from build123d import *

# Parameters (mm, degrees)
BOSS_EXTRUDE1_DEPTH = 30
SKETCH2_W           = 19.5
SKETCH2_H           = 19.5
BOSS_EXTRUDE2_DEPTH = 19.5
SKETCH3_W           = 55
SKETCH3_H           = 10
BOSS_EXTRUDE3_DEPTH = 2.5


with BuildPart() as part:
    # Sketch1 → Boss-Extrude1 (new body)
    with BuildSketch(Plane.XY):
        Polygon((12, 0), (12, 3), (5, 3), (5, 7), (50, 7), (50, 3), (43, 3), (43, 0), (55, 0), (55, 10), (0, 10), (0, 0), align=None)
    extrude(amount=BOSS_EXTRUDE1_DEPTH)

    # Sketch2 → Boss-Extrude2 (add)
    with BuildSketch(Plane(origin=(0, 10, 0), x_dir=(1, 0, 0), z_dir=(0, 1, 0))):
        with Locations((27.5, -15)):
            Rectangle(SKETCH2_W, SKETCH2_H)
    extrude(amount=BOSS_EXTRUDE2_DEPTH)

    # Sketch3 → Boss-Extrude3 (add)
    with BuildSketch(Plane(origin=(0, 0, 0), x_dir=(-1, 0, 0), z_dir=(0, 0, -1))):
        with Locations((-27.5, 5)):
            Rectangle(SKETCH3_W, SKETCH3_H)
    extrude(amount=BOSS_EXTRUDE3_DEPTH)


solid = part.part
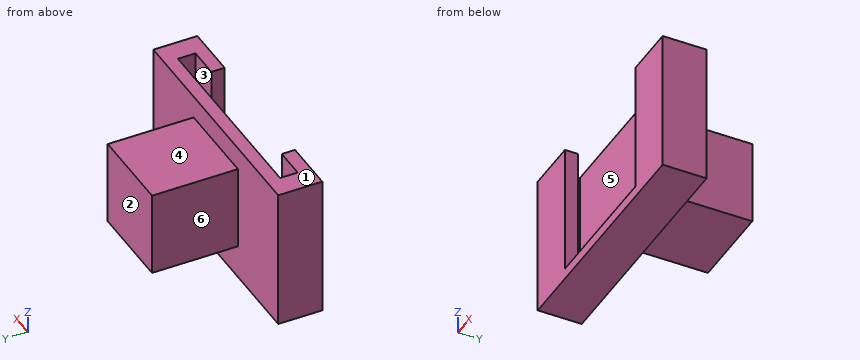
Read the model definition and answer for the solid it produces. Units are mm, in the model's axes. Face numbers are marked on the shaded views. A direction names the side the tool comes from. Round coordinates to 2 decimals unless told otherwise and drop trailing zeros. Write each loop counter-clockwise with the first axis right and the second up, starting at its lowest first coordinate (ties: lowest second). Pieces come first, ordered by that corner, then holes. Notation, with made-up numbers: (-24.5, 40.5) - (13.5, 40.5) arc R27 ccw to (13.5, 79.5) - close; hole circle Ø11 at (-9.75, 19). An arc over 180 degrees is marked (long way). Use a Markdown table: item, result.
(1) The part is cut by section A-A (x = 44). Write down the section's boundary in (y, z), then the cut area to 3 significant figures.
Reported:
| item | result |
|---|---|
| outline | (0, -2.5) - (10, -2.5) - (10, 30) - (7, 30) - (7, 0) - (3, 0) - (3, 30) - (0, 30) - close |
| area | 205 mm2 |
(2) Each of these flat-tipped pins is pushed along its axis until it touches: pin 1 Ø9 at (x, z) = (36, 20.5) entering from -Y; pin 2 Ø5.5 at (x, y) = (23, 2) entering from +Z; pin 3 Ø5 at (x, y) = (35.5, 18.5) entering from +Z. Where does it stop, or does it pass through?
Reported:
| item | result |
|---|---|
| pin 1 | y = 7 |
| pin 2 | z = 0 |
| pin 3 | z = 24.75 |
(3) The part is cut by section C-C (z = 4). Write down the section's boundary in (x, y).
Reported:
| item | result |
|---|---|
| outline | (0, 0) - (12, 0) - (12, 3) - (5, 3) - (5, 7) - (50, 7) - (50, 3) - (43, 3) - (43, 0) - (55, 0) - (55, 10) - (0, 10) - close |
(4) Which of the six approach directions +Z, -Z, +X, -X, +Y, -Y give full straight-line access (tool end or side, diameter ignored) to the marked faces 4, 5 and 6?
Reported:
| item | result |
|---|---|
| face 4 | +Z, +X, -X, +Y |
| face 5 | +Z |
| face 6 | +Z, -Z, -X, +Y |
(5) The mould has two halves that part along Y. Classify the marked faces 1, 2 and 3: released by +Y, released by -Y, zero draft, split by the parting line, or undercut.
Reported:
| item | result |
|---|---|
| face 1 | zero draft |
| face 2 | released by +Y |
| face 3 | undercut |
(6) Straight lines are drawn through the part: line 1 along X through (y, z) = (5.75, 16); line 2 along Y through (x, z) = (8, 1.5); line 3 along Y through (x, z) = (35, 8.5). For each, find the intervals that lie inside material, in ascending order. Write a range as [from, to].
Reported:
| item | result |
|---|---|
| line 1 | [0, 5], [50, 55] |
| line 2 | [0, 3], [7, 10] |
| line 3 | [7, 29.5] |
(7) The part is cut by section B-B (y = 4.25). Write down the section's boundary in (x, z), then the cut area to 4 significant figures.
Reported:
| item | result |
|---|---|
| outline | (0, -2.5) - (55, -2.5) - (55, 30) - (50, 30) - (50, 0) - (5, 0) - (5, 30) - (0, 30) - close |
| area | 437.5 mm2 |
(8) The part is cut by section D-D (x = 24). Write down the section's boundary in (y, z), then the cut area to 3 significant figures.
Reported:
| item | result |
|---|---|
| outline | (0, -2.5) - (10, -2.5) - (10, 5.25) - (29.5, 5.25) - (29.5, 24.75) - (10, 24.75) - (10, 30) - (7, 30) - (7, 0) - (0, 0) - close |
| area | 495 mm2 |
